Verification items for the finished model (mm, model axes). A direction names the side the tool comes from. Round coordinates to 2 decimals unless told otherwise and drop trailing zeros. Loops run counter-clockwise (first coordinate to the right, second up) from the corner with the lowest first, then second, coordinate; pieces in that order, holes last.
from build123d import *

# Parameters (mm, degrees)
F0_W     = 203.2
F0_H     = 152.4
F1_DEPTH = 71.12
F2_R     = 5.08
F3_T     = 5.08
F4_R     = 4
F5_DEPTH = 71.12
F7_D     = 4
F7_DEPTH = 25.4
F7_TIP   = 1.2017212381


# Not quite as in the source:
# - a shell that OpenCascade refuses in one call is made with other operations: the cavity is built on its own and cut out


with BuildPart() as f1:
    # F0 (on Front) → F1 (new body)
    with BuildSketch(Plane.XZ):
        with Locations((101.6, 76.2)):
            Rectangle(F0_W, F0_H)
    extrude(amount=F1_DEPTH)

    # F2
    f2_edges = [f1.edges().sort_by_distance(p)[0] for p in [
        (0, -35.56, 152.4),
        (0, -35.56, 0),
        (203.2, -35.56, 152.4),
        (203.2, -35.56, 0),
    ]]
    fillet(f2_edges, radius=F2_R)

    # F3: shell of thickness 5.08, made by hand


with BuildPart() as f3_core1:
    # F3_t2: copy of F1
    add(f1.part)

    # the walls: a layer under each face that stays
    f3_faces = [f3_core1.faces().sort_by_distance(p)[0] for p in [
        (0, -35.56, 76.2),
        (101.6, 0, 76.2),
        (101.6, -35.56, 152.4),
        (101.6, -35.56, 0),
        (203.2, -35.56, 76.2),
    ]]
    thicken(f3_faces, amount=-F3_T, mode=Mode.SUBTRACT)


with BuildPart() as f1_1:
    add(f1.part)

    # what is left inside the walls is the cavity
    f3_cavity = [f3_core1.part.solids().sort_by_distance(p)[0] for p in [
        (101.6, -5.1308, 52.493333),
    ]]
    add(f3_cavity, mode=Mode.SUBTRACT)

    # F4 (on Front) → F5 (join)
    with BuildSketch(Plane.XZ):
        with Locations((7.0729700904, 145.7453031343)):
            Circle(F4_R)
        with Locations((196.0783849807, 145.8089049954)):
            Circle(F4_R)
        with Locations((7.0786034794, 6.6475407913)):
            Circle(F4_R)
        with Locations((196.1331322956, 6.6623895618)):
            Circle(F4_R)
    extrude(amount=F5_DEPTH)

    # F7
    with Locations(Plane.XZ.offset(71.12)):
        with Locations((7.0729700904, 145.7453031343), (7.0786034794, 6.6475407913), (196.1331322956, 6.6623895618), (196.0783849807, 145.8089049954)):
            Hole(F7_D / 2, depth=F7_DEPTH)
            with Locations((0, 0, -(F7_DEPTH + F7_TIP / 2))):  # 118° drill point
                Cone(0, F7_D / 2, F7_TIP, mode=Mode.SUBTRACT)


solid = f1_1.part
1. Gauge pin test, flat ends, axial feed: P1, Ø3, axis at x = 196.08, z = 145.81, coming from the +Y side; P2, Ø6, axis at x = 161, z = 50, coming from the -Y side; P3, Ø3.5, axis at x = 7.07, z = 145.75, coming from the -Y side; P4, Ø3, axis at x = 196.13, z = 6.66, coming from the -Y side. Record the tip position at first contact, or that the pin passes through.
2. Scan lines: L1, parallel to X at y = -21, z = 65.5; L2, parallel to Z at x = 59, y = -21; L3, parallel to Y at x = 29.5, z = 86. Record each from-to range of solid material in increasing order.
3. Release check for a two-part mould opening along Z. For faces 3 (the face through (195.73, -44.73, 145.82)), 4 (the face through (195.786, -44.727, 6.678)), 5 (the face through (1.449, -36.058, 150.872)), 6 (the face through (0, -35, 75)) record: released by +Z, released by -Z, zero draft, split by the parting line, or undercut.
4. Section check A-A (y = -9). Enter the section's corners in (x, z).
5. Section check B-B (x = 137). Enter the section's corners in (y, z).
6. Section check D-D (y = -61). Enter the section's corners in (x, z), then the cut area to 4 significant figures.
7. Section check C-C (z = 47.5). Enter the section's corners in (x, y).
8. Tool access check on faces 1 (the face through (201.751, -36.058, 150.872)), 2 (the face through (7.33, -58.24, 147.73)). Record the directions out of +Z, -Z, +X, -X, +Y, -Y that give a thin tool (end or side, any length) a straight path to the whole face; none if there is none.
Taken from the geometry:
1. P1: stops at y = 0
1. P2: stops at y = -5.08
1. P3: stops at y = -45.57
1. P4: stops at y = -45.42
2. L1: x = 0 to 5.08, 198.12 to 203.2
2. L2: z = 0 to 5.08, 147.32 to 152.4
2. L3: y = -5.08 to 0
3. face 3: undercut
3. face 4: undercut
3. face 5: released by +Z
3. face 6: zero draft
4. outline: (0, 5.08) arc R5.08 ccw to (5.08, 0) - (198.12, 0) arc R5.08 ccw to (203.2, 5.08) - (203.2, 147.32) arc R5.08 ccw to (198.12, 152.4) - (5.08, 152.4) arc R5.08 ccw to (0, 147.32) - close; hole (5.08, 10.11) arc R4 cw to (10.76, 5.08) - (192.46, 5.08) arc R4 cw to (198.12, 10.13) - (198.12, 142.37) arc R4 cw to (192.37, 147.32) - (10.75, 147.32) arc R4 cw to (5.08, 142.28) - close
5. outline: (-71.12, 0) - (0, 0) - (0, 152.4) - (-71.12, 152.4) - (-71.12, 147.32) - (-5.08, 147.32) - (-5.08, 5.08) - (-71.12, 5.08) - close
6. outline: (0, 5.08) arc R5.08 ccw to (5.08, 0) - (198.12, 0) arc R5.08 ccw to (203.2, 5.08) - (203.2, 147.32) arc R5.08 ccw to (198.12, 152.4) - (5.08, 152.4) arc R5.08 ccw to (0, 147.32) - close; hole circle Ø4 at (7.07, 145.75); hole circle Ø4 at (7.08, 6.65); hole (5.08, 10.11) arc R4 cw to (10.76, 5.08) - (192.46, 5.08) arc R4 cw to (198.12, 10.13) - (198.12, 142.37) arc R4 cw to (192.37, 147.32) - (10.75, 147.32) arc R4 cw to (5.08, 142.28) - close; hole circle Ø4 at (196.08, 145.81); hole circle Ø4 at (196.13, 6.66)
6. area: 3,555 mm2
7. outline: (0, -71.12) - (5.08, -71.12) - (5.08, -5.08) - (198.12, -5.08) - (198.12, -71.12) - (203.2, -71.12) - (203.2, 0) - (0, 0) - close
8. face 1: +Z, +X, +Y, -Y
8. face 2: -Y
